Geometry check sheet. Reference: the model listing, model coordinates, mm. A direction names the side the tool comes from. Round coordinates to 2 decimals unless told otherwise and drop trailing zeros. Write each loop counter-clockwise with the first axis right and the second up, starting at its lowest first coordinate (ties: lowest second). Pieces come first, ordered by that corner, then holes. Notation, with made-up numbers: M 87.5,79 L 92.5,79 A19 cw 92.5,89 Z; hole C -25.75,31 d7. An arc over 180 degrees is marked long. Answer in a Markdown table with one row per item. Add a question column.
from build123d import *

# Parameters (mm, degrees)
F1_DEPTH      = 101.6
F2_W          = 38.1
F2_H          = 38.1
F3_DEPTH      = 44.451
F5_DEPTH      = 76.2
F6_W          = 50.8
F6_H          = 25.4
F7_DEPTH      = 107.951
F7_DEPTH_BACK = 107.951


with BuildPart() as f1:
    # F0 (on Front) → F1 (new body)
    with BuildSketch(Plane.XZ):
        with BuildLine():
            Line((107.95, 0), (-107.95, 0))
            Line((-107.95, 0), (-107.95, -25.4))
            Line((-107.95, -25.4), (-57.15, -25.4))
            Line((-57.15, -25.4), (-57.15, -44.45))
            Line((-57.15, -44.45), (-38.1, -44.45))
            Line((-38.1, -44.45), (-38.1, -38.1))
            ThreePointArc((-38.1, -38.1), (-34.3802561211, -29.1197438789), (-25.4, -25.4))
            Line((-25.4, -25.4), (25.4, -25.4))
            ThreePointArc((25.4, -25.4), (34.3802561211, -29.1197438789), (38.1, -38.1))
            Line((38.1, -38.1), (38.1, -44.45))
            Line((38.1, -44.45), (57.15, -44.45))
            Line((57.15, -44.45), (57.15, -25.4))
            Line((57.15, -25.4), (107.95, -25.4))
            Line((107.95, -25.4), (107.95, 0))
        make_face()
    extrude(amount=F1_DEPTH)

    # F2 (on face) → F3 (cut, through all)
    with BuildSketch(Plane.XY):
        with BuildLine():
            ThreePointArc((-107.95, -12.7), (-104.2302561211, -3.7197438789), (-95.25, 0))
            Line((-95.25, 0), (-107.95, 0))
            Line((-107.95, 0), (-107.95, -12.7))
        make_face()
        with BuildLine():
            ThreePointArc((-95.25, -101.6), (-104.2302561211, -97.8802561211), (-107.95, -88.9))
            Line((-107.95, -88.9), (-107.95, -101.6))
            Line((-107.95, -101.6), (-95.25, -101.6))
        make_face()
        with BuildLine():
            ThreePointArc((107.95, -88.9), (104.2302561211, -97.8802561211), (95.25, -101.6))
            Line((95.25, -101.6), (107.95, -101.6))
            Line((107.95, -101.6), (107.95, -88.9))
        make_face()
        with BuildLine():
            ThreePointArc((95.25, 0), (104.2302561211, -3.7197438789), (107.95, -12.7))
            Line((107.95, -12.7), (107.95, 0))
            Line((107.95, 0), (95.25, 0))
        make_face()
        with Locations((-88.9, -50.8)):
            Rectangle(F2_W, F2_H)
        with Locations((88.9, -50.8)):
            Rectangle(F2_W, F2_H)
    extrude(amount=-F3_DEPTH, mode=Mode.SUBTRACT)

    # F4 (on face) → F5 (join)
    with BuildSketch(Plane.XY):
        Polygon((-50.8, 0), (0, -101.6), (50.8, 0), align=None)
    extrude(amount=F5_DEPTH)

    # F6 (on Right) → F7 (cut, two sides)
    with BuildSketch(Plane.YZ) as f7_sk:
        with Locations((-76.2, 44.45)):
            Rectangle(F6_W, F6_H)
    extrude(amount=-F7_DEPTH, mode=Mode.SUBTRACT)
    extrude(f7_sk.sketch, amount=F7_DEPTH_BACK, mode=Mode.SUBTRACT)


solid = f1.part
Item 1: Section check C-C, the plane z = -5. Record the boundary of the cut face in (x, y), and give its area (3 significant figures).
Item 2: Section check D-D, the plane y = -47. Record the boundary of the cut face in (x, z).
Item 3: Access from +Z, -Z, +X, -X, +Y, -Y to the whole of each face (thin tool, end or side, straight path). Record for faces 1 (the flat face through (-66, -50, -25.4)), 2 (the flat face through (38.1, -50, -41)), 3 (the flat face through (30.7, -40.2, 37.6)), 4 (the flat face through (69.85, -51, -13)).
Item 4: Mould release check, pull along Z, two halves, no side actions. Record for faces 5 (the flat face through (107.95, -79, -13)), 6 (the flat face through (0, -50.8, 44)), 7 (the cylindrical face through (34.28, -50.09, -29.02)): +Z half, -Z half, draft (parallel to the pull), parting line (faces both ways), or undercut.
Item 5: Section check B-B, the plane y = -77. Record the boundary of the cut face in (x, z).
Item 6: Scan lines: probe 1 along Z at (x, y) = (20.5, -59.5); probe 2 along Z at (x, y) = (-77, -18.5); probe 3 along Z at (x, y) = (1.5, -16). Record each from-to range of solid material in increasing order. Write a range as from..to.
Item 7: Gauge pin test, flat ends, axial feed: pin 1 Ø6 at (x, y) = (-2.5, -31) entering from -Z; pin 2 Ø1.9 at (y, z) = (-54.5, -42) entering from -X; pin 3 Ø1.5 at (y, z) = (-54.5, -30) entering from +X. Record the tip position at first contact, or that the pin passes through.
Item 8: Section check A-A, the plane x = -74. Record the boundary of the cut face in (y, z).
Result sheet:
| question | item | result |
|---|---|---|
| 1 | outline | M -107.95,-88.9 A12.7 ccw -95.25,-101.6 L 95.25,-101.6 A12.7 ccw 107.95,-88.9 L 107.95,-69.85 L 69.85,-69.85 L 69.85,-31.75 L 107.95,-31.75 L 107.95,-12.7 A12.7 ccw 95.25,0 L -95.25,0 A12.7 ccw -107.95,-12.7 L -107.95,-31.75 L -69.85,-31.75 L -69.85,-69.85 L -107.95,-69.85 Z |
| 1 | area | 18,900 mm^2 |
| 2 | outline | M -69.85,-25.4 L -57.15,-25.4 L -57.15,-44.45 L -38.1,-44.45 L -38.1,-38.1 A12.7 cw -25.4,-25.4 L 25.4,-25.4 A12.7 cw 38.1,-38.1 L 38.1,-44.45 L 57.15,-44.45 L 57.15,-25.4 L 69.85,-25.4 L 69.85,0 L 27.3,0 L 27.3,76.2 L -27.3,76.2 L -27.3,0 L -69.85,0 Z |
| 3 | face 1 | -Z, -X, +Y, -Y |
| 3 | face 2 | -Z, +Y, -Y |
| 3 | face 3 | +Z, +X, -Y |
| 3 | face 4 | +Z, -Z, +X |
| 4 | face 5 | draft |
| 4 | face 6 | undercut |
| 4 | face 7 | -Z half |
| 5 | outline | M -107.95,-25.4 L -57.15,-25.4 L -57.15,-44.45 L -38.1,-44.45 L -38.1,-38.1 A12.7 cw -25.4,-25.4 L 25.4,-25.4 A12.7 cw 38.1,-38.1 L 38.1,-44.45 L 57.15,-44.45 L 57.15,-25.4 L 107.95,-25.4 L 107.95,0 L 12.3,0 L 12.3,31.75 L -12.3,31.75 L -12.3,0 L -107.95,0 Z; M -12.3,57.15 L 12.3,57.15 L 12.3,76.2 L -12.3,76.2 Z |
| 6 | probe 1 | z = -25.4..31.75, 57.15..76.2 |
| 6 | probe 2 | z = -25.4..0 |
| 6 | probe 3 | z = -25.4..76.2 |
| 7 | pin 1 | stops at z = -25.4 |
| 7 | pin 2 | stops at x = -57.15 |
| 7 | pin 3 | stops at x = 57.15 |
| 8 | outline | M -101.6,-25.4 L -69.85,-25.4 L -69.85,0 L -101.6,0 Z; M -31.75,-25.4 L 0,-25.4 L 0,0 L -31.75,0 Z |
